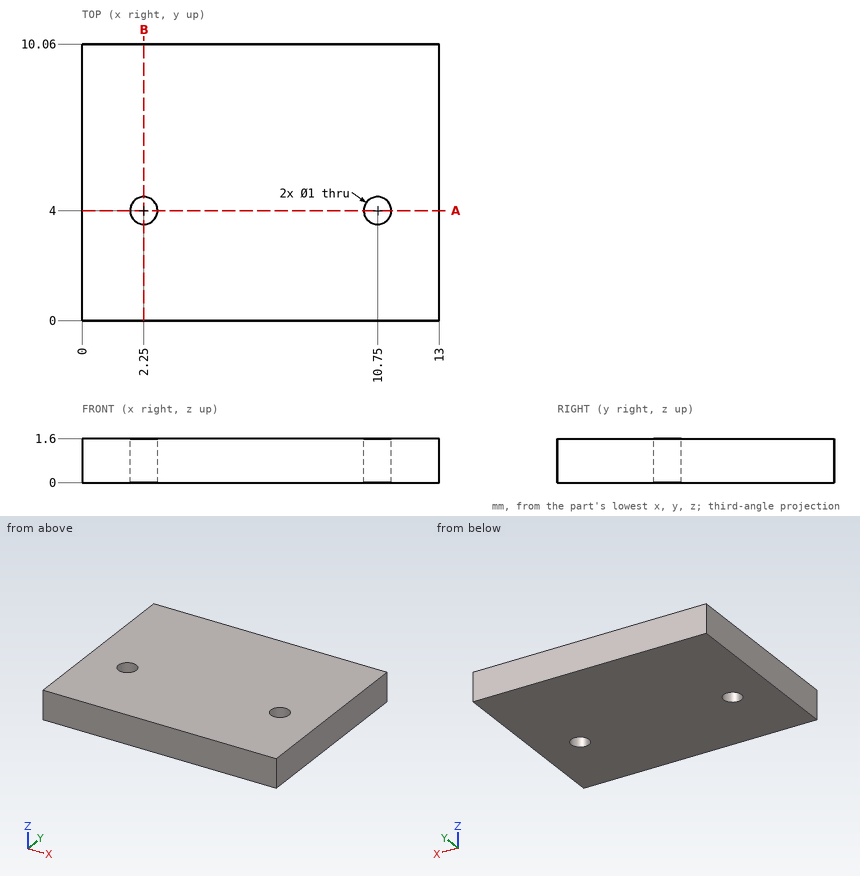
Design review of the part shown in the three views and the two pictorial views. Dimensions are in mm from the part's minimum x, y and z. Give positions to 0.01 mm unless a question says otherwise; leave off trailing zeros. Write each loop counter-clockwise with the first axis right and the second up, starting at its lowest first coordinate (ties: lowest second). Pieces come first, ordered by that corner, then holes. Notation, with made-up numbers: M 79,50.5 L 95,50.5 A25 ccw 95,73.5 Z; hole C -26.5,58.25 d2. An arc over 180 degrees is marked long. Return JSON: item names as keys, results as strings. Group by question number.
Item 1: Wall thickness on line 1 along X through (y, z) = (4, 0.5); line 2 along Y through (x, z) = (2.25, 1.15); line 3 along Y through (x, z) = (10.5, 0.75): over which ranges is each line inside the solid? List them lowest first.
Item 2: Take a section at B-B (x = 2.25). Give the boundary of the cut face in (y, z), plus the area to 3 significant figures.
Item 3: Take a section at A-A (y = 4). Give the boundary of the cut face in (x, z), plus the area to 3 significant figures.
Return value:
{
 "1": {"line 1": "x = 0 to 1.75, 2.75 to 10.25, 11.25 to 13", "line 2": "y = 0 to 3.5, 4.5 to 10.06", "line 3": "y = 0 to 3.57, 4.43 to 10.06"},
 "2": {"outline": "M 0,0 L 3.5,0 L 3.5,1.6 L 0,1.6 Z; M 4.5,0 L 10.06,0 L 10.06,1.6 L 4.5,1.6 Z", "area": "14.5 mm2"},
 "3": {"outline": "M 0,0 L 1.75,0 L 1.75,1.6 L 0,1.6 Z; M 2.75,0 L 10.25,0 L 10.25,1.6 L 2.75,1.6 Z; M 11.25,0 L 13,0 L 13,1.6 L 11.25,1.6 Z", "area": "17.6 mm2"}
}
